Could you check a few things on this model? Use its own coordinates, in mm. Coordinates: 2 decimals unless noted, no trailing zeros. Write each loop counter-clockwise with the first axis right and the second up, starting at its lowest first coordinate (ties: lowest second). Pieces come first, ordered by that corner, then holes. Notation, with made-up numbers: M 21.25,-30.5 L 75.25,-30.5 A14 ccw 75.25,-18.5 Z; hole C -9,-19.5 d5. An arc over 180 degrees is marked long. Answer as CSV lines item,"result". Start each with the question number.
Item 1: If I drill on line 1 along Z through (x, y) = (0, -1.4); line 2 along X through (y, z) = (-0.75, 0.5); line 3 along Z through (x, y) = (-1, -1.65), over which ranges is the centre line in solid material (lowest first)? Write a range as [from, to].
Item 2: I'm going to push a flat-ended pin straight in: P1, Ø1, axis at x = 7, y = -0.5, coming from the +Z side. Where does the tip first touch, or does it pass through?
Item 3: Suppose I cut it at A-A, the plane x = 0. Write out the boundary of the cut face in (y, z).
Item 4: Suppose I cut it at B-B, the plane z = 0. Write out the boundary of the cut face in (x, y), and give its area (3 significant figures).
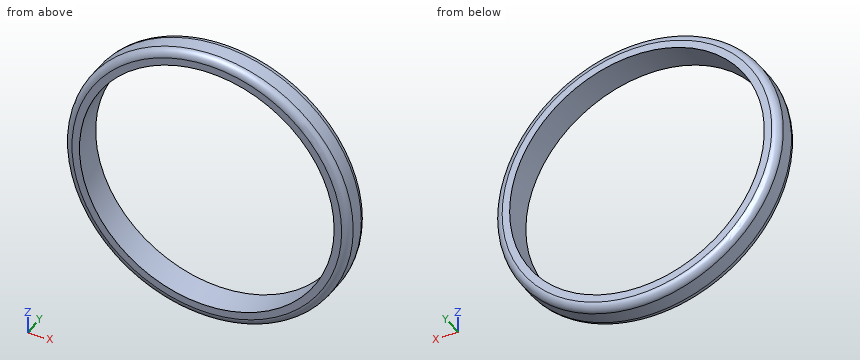
```python
from build123d import *

# Parameters (mm, degrees)
F0_R     = 9.5
F1_DEPTH = 2
F2_R     = 8.5
F3_DEPTH = 2.001
F4_R     = 0.5


with BuildPart() as f1:
    # F0 (on Front) → F1 (new body)
    with BuildSketch(Plane.XZ):
        Circle(F0_R)
    extrude(amount=F1_DEPTH)

    # F2 (on face) → F3 (cut, through all)
    with BuildSketch(Plane.XZ.offset(2)):
        Circle(F2_R)
    extrude(amount=-F3_DEPTH, mode=Mode.SUBTRACT)

    # F4
    f4_edges = [f1.edges().sort_by_distance(p)[0] for p in [
        (-9.5, -2, 0),
        (-9.5, 0, 0),
    ]]
    fillet(f4_edges, radius=F4_R)


solid = f1.part
```
Ans:
1,line 1,"z = [-9.5, -8.5], [8.5, 9.5]"
1,line 2,"x = [-9.49, -8.49], [8.49, 9.49]"
1,line 3,"z = [-9.42, -8.44], [8.44, 9.42]"
2,P1,"stops at z = 6.93"
3,outline,"M -2,-9 A0.5 ccw -1.5,-9.5 L -0.5,-9.5 A0.5 ccw 0,-9 L 0,-8.5 L -2,-8.5 Z; M -2,8.5 L 0,8.5 L 0,9 A0.5 ccw -0.5,9.5 L -1.5,9.5 A0.5 ccw -2,9 Z"
4,outline,"M -9.5,-1.5 A0.5 ccw -9,-2 L -8.5,-2 L -8.5,0 L -9,0 A0.5 ccw -9.5,-0.5 Z; M 8.5,-2 L 9,-2 A0.5 ccw 9.5,-1.5 L 9.5,-0.5 A0.5 ccw 9,0 L 8.5,0 Z"
4,area,"3.79 mm^2"
